from build123d import *

# Parameters (mm, degrees)
F1_DEPTH  = 0.5
F1_FACE_W = 1
F1_FACE_H = 3
F6_DEPTH  = 5
F8_DEPTH  = 25


# Not quite as in the source:
# - the arcs of a loft's sections are written as splines that run evenly, so that the points pair up as in the source's solid


with BuildPart() as f1:
    # F0 (on Front) → F1 (new body, symmetric)
    with BuildSketch(Plane.XZ):
        Polygon((-0.0253911159, 2.9998925466), (0, 0), (50, 0), (49.8984355364, 11.9995701865), (14.899088368, 11.7857997863), align=None)
    extrude(amount=F1_DEPTH, both=True)

    # F1_face (on face) → F4 section 0
    with BuildSketch(Plane(origin=(-0.0126955579, 0, 1.4999462733), x_dir=(0, -1, 0), z_dir=(-0.9999641822, 0, -0.0084637053))):
        Rectangle(F1_FACE_W, F1_FACE_H)
    # F3 (on offset) → F4 section 1
    with BuildSketch(Plane.YZ.offset(-3)):
        with BuildLine():
            add(Edge.make_bspline(
                [(-0.4743722327, 2.9230147522), (-0.6606444281, 2.8609195721), (-0.834496694, 2.7618115588), (-1.1311572384, 2.5045080607), (-1.2538487938, 2.3464138139), (-1.4294616132, 1.995169303), (-1.482313781, 1.8021572386), (-1.5101434154, 1.4104455076), (-1.4851099322, 1.2118999628), (-1.4230147522, 1.0256277673)],
                knots=[0, 0, 0, 0, 0.25, 0.25, 0.5, 0.5, 0.75, 0.75, 1, 1, 1, 1], degree=3))
            add(Edge.make_bspline(
                [(-1.4230147522, 1.0256277673), (-1.3609195721, 0.8393555719), (-1.2618115588, 0.665503306), (-1.0045080607, 0.3688427616), (-0.8464138139, 0.2461512062), (-0.495169303, 0.0705383868), (-0.3021572386, 0.017686219), (0.0895544924, -0.0101434154), (0.2881000372, 0.0148900678), (0.4743722327, 0.0769852478)],
                knots=[0, 0, 0, 0, 0.25, 0.25, 0.5, 0.5, 0.75, 0.75, 1, 1, 1, 1], degree=3))
            add(Edge.make_bspline(
                [(0.4743722327, 0.0769852478), (0.6606444281, 0.1390804279), (0.834496694, 0.2381884412), (1.1311572384, 0.4954919393), (1.2538487938, 0.6535861861), (1.4294616132, 1.004830697), (1.482313781, 1.1978427614), (1.5101434154, 1.5895544924), (1.4851099322, 1.7881000372), (1.4230147522, 1.9743722327)],
                knots=[0, 0, 0, 0, 0.25, 0.25, 0.5, 0.5, 0.75, 0.75, 1, 1, 1, 1], degree=3))
            add(Edge.make_bspline(
                [(1.4230147522, 1.9743722327), (1.3609195721, 2.1606444281), (1.2618115588, 2.334496694), (1.0045080607, 2.6311572384), (0.8464138139, 2.7538487938), (0.495169303, 2.9294616132), (0.3021572386, 2.982313781), (-0.0895544924, 3.0101434154), (-0.2881000372, 2.9851099322), (-0.4743722327, 2.9230147522)],
                knots=[0, 0, 0, 0, 0.25, 0.25, 0.5, 0.5, 0.75, 0.75, 1, 1, 1, 1], degree=3))
        make_face()
    loft(ruled=True)

    # F5 (on face) → F6 (join)
    with BuildSketch(Plane(origin=(-3, 0, 0), x_dir=(0, -1, 0), z_dir=(-1, 0, 0))):
        with BuildLine():
            add(Edge.make_bspline(
                [(0.2236067977, 0.9472135955), (0.2049485822, 0.9590404276), (0.165567887, 0.9783654777), (0.1016629971, 0.9971413164), (0.0354857267, 0.9971906029), (-0.0298581595, 1.006417373), (-0.0962378171, 0.9979647462), (-0.1574135127, 0.9730184068), (-0.2213803356, 0.9564199077), (-0.2794920021, 0.9232440711), (-0.3264257064, 0.8766967879), (-0.3795448144, 0.8369923373), (-0.419371865, 0.7835849556), (-0.4393276132, 0.744366395), (-0.4472135955, 0.7236067977)],
                knots=[0, 0, 0, 0, 0.0661130278, 0.1311431351, 0.1976238463, 0.263561262, 0.3285913694, 0.3952621183, 0.461199534, 0.5262296414, 0.5929003903, 0.6590289395, 0.7240590469, 0.7905532518, 0.7905532518, 0.7905532518, 0.7905532518], degree=3))
            add(Edge.make_bspline(
                [(-0.4472135955, 0.7236067977), (-0.4590404276, 0.7049485822), (-0.4783654777, 0.665567887), (-0.4971413164, 0.6016629971), (-0.4971906029, 0.5354857267), (-0.506417373, 0.4701418405), (-0.4979647462, 0.4037621829), (-0.4730184068, 0.3425864873), (-0.4564199077, 0.2786196644), (-0.4232440711, 0.2205079979), (-0.3766967879, 0.1735742936), (-0.3369923373, 0.1204551856), (-0.2835849556, 0.080628135), (-0.244366395, 0.0606723868), (-0.2236067977, 0.0527864045)],
                knots=[0, 0, 0, 0, 0.0661130278, 0.1311431351, 0.1976238463, 0.263561262, 0.3285913694, 0.3952621183, 0.461199534, 0.5262296414, 0.5929003903, 0.6590289395, 0.7240590469, 0.7905532518, 0.7905532518, 0.7905532518, 0.7905532518], degree=3))
            add(Edge.make_bspline(
                [(-0.2236067977, 0.0527864045), (-0.2049485822, 0.0409595724), (-0.165567887, 0.0216345223), (-0.1016629971, 0.0028586836), (-0.0533041533, 0.0028226676), (-0.0269411852, 0.0005980705), (-0.0226951286, 0.0002149422)],
                knots=[0, 0, 0, 0, 0.0661130278, 0.1311431351, 0.1976238463, 0.2103977386, 0.2103977386, 0.2103977386, 0.2103977386], degree=3))
            add(Edge.make_bspline(
                [(0.0857219406, 0.0024530962), (0.0496252148, 0.0003925316), (0.0134550487, -0.000349593), (-0.0226951286, 0.0002149422)],
                knots=[0.7587522631, 0.7587522631, 0.7587522631, 0.7587522631, 0.8047879331, 0.8047879331, 0.8047879331, 0.8047879331], degree=3))
            add(Edge.make_bspline(
                [(0.0857219406, 0.0024530962), (0.0887772594, 0.0031276832), (0.1134683814, 0.0090615655), (0.1574135127, 0.0269815932), (0.2213803356, 0.0435800923), (0.2794920021, 0.0767559289), (0.3264257064, 0.1233032121), (0.3795448144, 0.1630076627), (0.419371865, 0.2164150444), (0.4393276132, 0.255633605), (0.4472135955, 0.2763932023)],
                knots=[0.3192274693, 0.3192274693, 0.3192274693, 0.3192274693, 0.3285913694, 0.3952621183, 0.461199534, 0.5262296414, 0.5929003903, 0.6590289395, 0.7240590469, 0.7905532518, 0.7905532518, 0.7905532518, 0.7905532518], degree=3))
            add(Edge.make_bspline(
                [(0.4472135955, 0.2763932023), (0.4590404276, 0.2950514178), (0.4783654777, 0.334432113), (0.4971413164, 0.3983370029), (0.4971906029, 0.4645142733), (0.506417373, 0.5298581595), (0.4979647462, 0.5962378171), (0.4730184068, 0.6574135127), (0.4564199077, 0.7213803356), (0.4232440711, 0.7794920021), (0.3766967879, 0.8264257064), (0.3369923373, 0.8795448144), (0.2835849556, 0.919371865), (0.244366395, 0.9393276132), (0.2236067977, 0.9472135955)],
                knots=[0, 0, 0, 0, 0.0661130278, 0.1311431351, 0.1976238463, 0.263561262, 0.3285913694, 0.3952621183, 0.461199534, 0.5262296414, 0.5929003903, 0.6590289395, 0.7240590469, 0.7905532518, 0.7905532518, 0.7905532518, 0.7905532518], degree=3))
        make_face()
        with BuildLine():
            add(Edge.make_bspline(
                [(-0.4472135955, 0.7236067977), (-0.4590404276, 0.7049485822), (-0.4783654777, 0.665567887), (-0.4971413164, 0.6016629971), (-0.4971906029, 0.5354857267), (-0.506417373, 0.4701418405), (-0.4979647462, 0.4037621829), (-0.4730184068, 0.3425864873), (-0.4564199077, 0.2786196644), (-0.4232440711, 0.2205079979), (-0.3766967879, 0.1735742936), (-0.3369923373, 0.1204551856), (-0.2835849556, 0.080628135), (-0.244366395, 0.0606723868), (-0.2236067977, 0.0527864045)],
                knots=[0, 0, 0, 0, 0.0661130278, 0.1311431351, 0.1976238463, 0.263561262, 0.3285913694, 0.3952621183, 0.461199534, 0.5262296414, 0.5929003903, 0.6590289395, 0.7240590469, 0.7905532518, 0.7905532518, 0.7905532518, 0.7905532518], degree=3))
            add(Edge.make_bspline(
                [(0.2236067977, 0.9472135955), (0.2049485822, 0.9590404276), (0.165567887, 0.9783654777), (0.1016629971, 0.9971413164), (0.0354857267, 0.9971906029), (-0.0298581595, 1.006417373), (-0.0962378171, 0.9979647462), (-0.1574135127, 0.9730184068), (-0.2213803356, 0.9564199077), (-0.2794920021, 0.9232440711), (-0.3264257064, 0.8766967879), (-0.3795448144, 0.8369923373), (-0.419371865, 0.7835849556), (-0.4393276132, 0.744366395), (-0.4472135955, 0.7236067977)],
                knots=[0, 0, 0, 0, 0.0661130278, 0.1311431351, 0.1976238463, 0.263561262, 0.3285913694, 0.3952621183, 0.461199534, 0.5262296414, 0.5929003903, 0.6590289395, 0.7240590469, 0.7905532518, 0.7905532518, 0.7905532518, 0.7905532518], degree=3))
            add(Edge.make_bspline(
                [(0.4472135955, 0.2763932023), (0.4590404276, 0.2950514178), (0.4783654777, 0.334432113), (0.4971413164, 0.3983370029), (0.4971906029, 0.4645142733), (0.506417373, 0.5298581595), (0.4979647462, 0.5962378171), (0.4730184068, 0.6574135127), (0.4564199077, 0.7213803356), (0.4232440711, 0.7794920021), (0.3766967879, 0.8264257064), (0.3369923373, 0.8795448144), (0.2835849556, 0.919371865), (0.244366395, 0.9393276132), (0.2236067977, 0.9472135955)],
                knots=[0, 0, 0, 0, 0.0661130278, 0.1311431351, 0.1976238463, 0.263561262, 0.3285913694, 0.3952621183, 0.461199534, 0.5262296414, 0.5929003903, 0.6590289395, 0.7240590469, 0.7905532518, 0.7905532518, 0.7905532518, 0.7905532518], degree=3))
            add(Edge.make_bspline(
                [(0.0857219406, 0.0024530962), (0.0887772594, 0.0031276832), (0.1134683814, 0.0090615655), (0.1574135127, 0.0269815932), (0.2213803356, 0.0435800923), (0.2794920021, 0.0767559289), (0.3264257064, 0.1233032121), (0.3795448144, 0.1630076627), (0.419371865, 0.2164150444), (0.4393276132, 0.255633605), (0.4472135955, 0.2763932023)],
                knots=[0.3192274693, 0.3192274693, 0.3192274693, 0.3192274693, 0.3285913694, 0.3952621183, 0.461199534, 0.5262296414, 0.5929003903, 0.6590289395, 0.7240590469, 0.7905532518, 0.7905532518, 0.7905532518, 0.7905532518], degree=3))
            add(Edge.make_bspline(
                [(1.4230147522, 1.0256277673), (1.3609195721, 0.8393555719), (1.2618115588, 0.665503306), (1.0045080607, 0.3688427616), (0.8464138139, 0.2461512062), (0.495169303, 0.0705383868), (0.3021572386, 0.017686219), (0.0994446448, 0.0032842572), (0.09258462, 0.002844849), (0.0857219406, 0.0024530962)],
                knots=[0, 0, 0, 0, 0.25, 0.25, 0.5, 0.5, 0.75, 0.75, 0.7587522631, 0.7587522631, 0.7587522631, 0.7587522631], degree=3))
            add(Edge.make_bspline(
                [(0.4743722327, 2.9230147522), (0.6606444281, 2.8609195721), (0.834496694, 2.7618115588), (1.1311572384, 2.5045080607), (1.2538487938, 2.3464138139), (1.4294616132, 1.995169303), (1.482313781, 1.8021572386), (1.5101434154, 1.4104455076), (1.4851099322, 1.2118999628), (1.4230147522, 1.0256277673)],
                knots=[0, 0, 0, 0, 0.25, 0.25, 0.5, 0.5, 0.75, 0.75, 1, 1, 1, 1], degree=3))
            add(Edge.make_bspline(
                [(-1.4230147522, 1.9743722327), (-1.3609195721, 2.1606444281), (-1.2618115588, 2.334496694), (-1.0045080607, 2.6311572384), (-0.8464138139, 2.7538487938), (-0.495169303, 2.9294616132), (-0.3021572386, 2.982313781), (0.0895544924, 3.0101434154), (0.2881000372, 2.9851099322), (0.4743722327, 2.9230147522)],
                knots=[0, 0, 0, 0, 0.25, 0.25, 0.5, 0.5, 0.75, 0.75, 1, 1, 1, 1], degree=3))
            add(Edge.make_bspline(
                [(-0.4743722327, 0.0769852478), (-0.6606444281, 0.1390804279), (-0.834496694, 0.2381884412), (-1.1311572384, 0.4954919393), (-1.2538487938, 0.6535861861), (-1.4294616132, 1.004830697), (-1.482313781, 1.1978427614), (-1.5101434154, 1.5895544924), (-1.4851099322, 1.7881000372), (-1.4230147522, 1.9743722327)],
                knots=[0, 0, 0, 0, 0.25, 0.25, 0.5, 0.5, 0.75, 0.75, 1, 1, 1, 1], degree=3))
            add(Edge.make_bspline(
                [(-0.0226951286, 0.0002149422), (-0.1759882345, 0.002608827), (-0.3289219115, 0.0284983341), (-0.4743722327, 0.0769852478)],
                knots=[0.8047879331, 0.8047879331, 0.8047879331, 0.8047879331, 1, 1, 1, 1], degree=3))
            add(Edge.make_bspline(
                [(-0.2236067977, 0.0527864045), (-0.2049485822, 0.0409595724), (-0.165567887, 0.0216345223), (-0.1016629971, 0.0028586836), (-0.0533041533, 0.0028226676), (-0.0269411852, 0.0005980705), (-0.0226951286, 0.0002149422)],
                knots=[0, 0, 0, 0, 0.0661130278, 0.1311431351, 0.1976238463, 0.2103977386, 0.2103977386, 0.2103977386, 0.2103977386], degree=3))
        make_face()
    extrude(amount=F6_DEPTH)

    # F7 (on face) → F8 (cut)
    with BuildSketch(Plane.XZ.offset(0.5)):
        Polygon((49.8984355364, 11.9995701865), (47.6442072011, 11.9858017213), (49.9094060968, 10.7034277653), align=None)
    extrude(amount=-F8_DEPTH, mode=Mode.SUBTRACT)


solid = f1.part
For this review, take the finished solid that the model builds, in its own axes (mm). A direction names the side the tool comes from. Round coordinates to 2 decimals unless told otherwise and drop trailing zeros. Order: outer loops, then holes, each group sorted by start corner. A loop starts at its lowest first (then second) coordinate and runs counter-clockwise, first axis right, second up. Notation, with made-up numbers: M 67,49 L 107,49 A33 ccw 107,88 Z; hole C 39,-21 d10. An arc over 180 degrees is marked long. Use a Markdown table: item, result. Add a question column.
Item 1: Insertion check: pin 1 (6 mm diameter, centred on x = 36.5, z = 8, fed in from -Y); pin 2 (3.5 mm diameter, centred on x = 21.5, z = 5.5, fed in from +Y). Each pin has a flat end and moves straight along its axis. Give the tip position at first contact, or say it passes through.
Item 2: Add section B-B, the plane x = 34.5. Give the boundary of the cut face in (y, z), then the cut area to 3 significant figures.
Item 3: Tool access review of faces 1 (the flat face through (25, 0.5, 6)), 2 (the flat face through (25, -0.5, 6)), 3 (the flat face through (7.541, -0.007, 7.454)): name each direction out of +Z, -Z, +X, -X, +Y, -Y from which nothing blocks a thin tool from reaching the whole face with its end or side.
Item 4: To check wall thickness, follow line 1 along Y through (x, z) = (1, 2); line 2 along Z through (x, y) = (17, 0.3); line 3 along X through (y, z) = (0.1, 1.5). State the ranges of each line that lie inside material, in increasing order.
Item 5: Add section A-A, the plane z = 5.25. Give the boundary of the cut face in (x, y), then the cut area to 3 significant figures.
Geometry results:
| question | item | result |
|---|---|---|
| 1 | pin 1 | stops at y = -0.5 |
| 1 | pin 2 | stops at y = 0.5 |
| 2 | outline | M -0.5,0 L 0.5,0 L 0.5,11.91 L -0.5,11.91 Z |
| 2 | area | 11.9 mm² |
| 3 | face 1 | +Z, -Z, +X, +Y |
| 3 | face 2 | +Z, -Z, +X, -Y |
| 3 | face 3 | +Z, -X, +Y, -Y |
| 4 | line 1 | y = -0.5 to 0.5 |
| 4 | line 2 | z = 0 to 11.8 |
| 4 | line 3 | x = -8 to 49.99 |
| 5 | outline | M 3.8,-0.5 L 49.96,-0.5 L 49.96,0.5 L 3.8,0.5 Z |
| 5 | area | 46.2 mm² |
